Input: part model. Units: mm. Frame: model coordinates. Face numbers are marked on the shaded views. A direction names the side the tool comes from. Coordinates: 2 decimals unless noted, no trailing zeros. Loops run counter-clockwise (first coordinate to the right, second up) from the corner with the lowest first, then second, coordinate; pieces in that order, holes last.
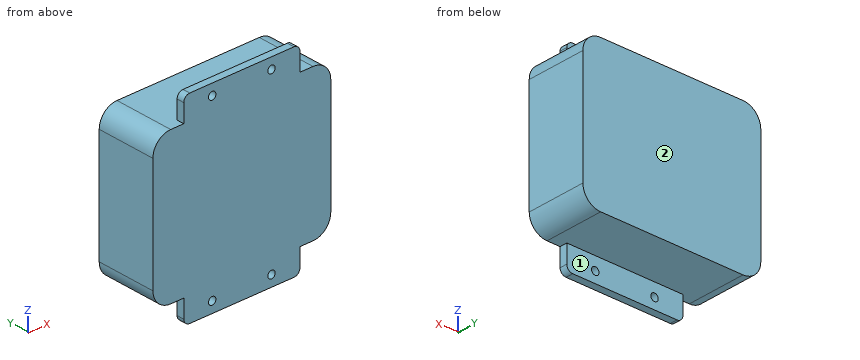
```python
from build123d import *

# Parameters (mm, degrees)
BOSS_EXTRUDE1_DEPTH = 25.4
SKETCH2_R           = 1.5875
BOSS_EXTRUDE2_DEPTH = 3.175


with BuildPart() as part:
    # Sketch1 → Boss-Extrude1 (new body)
    with BuildSketch(Plane(origin=(0, 0, 0), x_dir=(1, 0, 0), z_dir=(0, 1, 0))):
        with BuildLine():
            Line((-30.48, -31.75), (30.48, -31.75))
            ThreePointArc((30.48, -31.75), (35.868153673, -29.518153673), (38.1, -24.13))
            Line((38.1, -24.13), (38.1, 24.13))
            ThreePointArc((38.1, 24.13), (35.868153673, 29.518153673), (30.48, 31.75))
            Line((30.48, 31.75), (-30.48, 31.75))
            ThreePointArc((-30.48, 31.75), (-35.868153673, 29.518153673), (-38.1, 24.13))
            Line((-38.1, 24.13), (-38.1, -24.13))
            ThreePointArc((-38.1, -24.13), (-35.868153673, -29.518153673), (-30.48, -31.75))
        make_face()
    extrude(amount=BOSS_EXTRUDE1_DEPTH)

    # Sketch2 → Boss-Extrude2 (add)
    with BuildSketch(Plane(origin=(0, 0, 0), x_dir=(1, 0, 0), z_dir=(0, 1, 0))):
        with BuildLine():
            Line((-24.869490834, -31.75), (24.869490834, -31.75))
            Line((24.869490834, -31.75), (24.869490834, -39.431167642))
            ThreePointArc((24.869490834, -39.431167642), (24.125542058, -41.227218866), (22.329490834, -41.971167642))
            Line((22.329490834, -41.971167642), (-22.329490834, -41.971167642))
            ThreePointArc((-22.329490834, -41.971167642), (-24.125542058, -41.227218866), (-24.869490834, -39.431167642))
            Line((-24.869490834, -39.431167642), (-24.869490834, -31.75))
        make_face()
        with Locations((12.7, -37.35)):
            Circle(SKETCH2_R, mode=Mode.SUBTRACT)
        with Locations((-12.7, -37.35)):
            Circle(SKETCH2_R, mode=Mode.SUBTRACT)
        with BuildLine():
            Line((-24.869490834, 31.75), (-24.869490834, 39.431167642))
            ThreePointArc((-24.869490834, 39.431167642), (-24.125542058, 41.227218866), (-22.329490834, 41.971167642))
            Line((-22.329490834, 41.971167642), (22.329490834, 41.971167642))
            ThreePointArc((22.329490834, 41.971167642), (24.125542058, 41.227218866), (24.869490834, 39.431167642))
            Line((24.869490834, 39.431167642), (24.869490834, 31.75))
            Line((24.869490834, 31.75), (-24.869490834, 31.75))
        make_face()
        with Locations((12.7, 37.35)):
            Circle(SKETCH2_R, mode=Mode.SUBTRACT)
        with Locations((-12.7, 37.35)):
            Circle(SKETCH2_R, mode=Mode.SUBTRACT)
    extrude(amount=BOSS_EXTRUDE2_DEPTH)


solid = part.part
```
Item 1: Reachability of the marked faces 1 and 2 from +Z, -Z, +X, -X, +Y, -Y: full face, straight path, thin tool, end or side. Return the list, or none.
Result:
face 1: -Z, +X, -X, +Y
face 2: +Z, -Z, +X, -X, +Y
Item 2: Section query B-B (z = -37.35). Output: boundary loops of the cut face in (x, y) (1 decimal), then the cut area to 3 significant figures.
Result:
outline: (-24.9, 0) - (-14.3, 0) - (-14.3, 3.2) - (-24.9, 3.2) - close; (-11.1, 0) - (11.1, 0) - (11.1, 3.2) - (-11.1, 3.2) - close; (14.3, 0) - (24.9, 0) - (24.9, 3.2) - (14.3, 3.2) - close
area: 138 mm2
Item 3: Section query D-D (x = -8.5). Output: boundary loops of the cut face in (y, z) (3 decimals), then the cut area to 3 significant figures.
Result:
outline: (0, -41.971) - (3.175, -41.971) - (3.175, -31.75) - (25.4, -31.75) - (25.4, 31.75) - (3.175, 31.75) - (3.175, 41.971) - (0, 41.971) - close
area: 1,680 mm2
Item 4: Contact query for flat-ended pins moving along their axis: P1, Ø1, axis at y = 2, z = 34, coming from the +X side; P2, Ø1, axis at x = 17, y = 16, coming from the -Z side; P3, Ø4, axis at x = 12.7, z = 37.35, coming from the +Y side (3 decimals); P4, Ø1.9, axis at x = -12.7, z = 37.35, coming from the -Y side. Output: stop coordinate, or through.
Result:
P1: stops at x = 24.87
P2: stops at z = -31.75
P3: stops at y = 3.175
P4: passes through
Item 5: Line query: L1, parallel to Z at x = 12.7, y = 1.3; L2, parallel to X at y = 2, z = -37.35; L3, parallel to Z at x = -28.5, y = 9.75. Output: solid intervals per line, ascending.
Result:
L1: z = -41.97 to -38.94, -35.76 to 35.76, 38.94 to 41.97
L2: x = -24.87 to -14.29, -11.11 to 11.11, 14.29 to 24.87
L3: z = -31.75 to 31.75
Item 6: Section query A-A (x = 12.7). Count the separate pieces of the cut face and the enclosed holes in it, then the cut area to 3 significant figures.
Result:
separate pieces: 3
enclosed holes: 0
area: 1,660 mm2
Item 7: Section query C-C (y = 22). Output: boundary loops of the cut face in (x, z).
Result:
outline: (-38.1, -24.13) arc R7.62 ccw to (-30.48, -31.75) - (30.48, -31.75) arc R7.62 ccw to (38.1, -24.13) - (38.1, 24.13) arc R7.62 ccw to (30.48, 31.75) - (-30.48, 31.75) arc R7.62 ccw to (-38.1, 24.13) - close
